Autodesk Inventor part; units mm, degrees
ref_plane "YZ Plane" through (0, 0, 0) normal (1, 0, 0) x (0, 1, 0)
ref_plane "XZ Plane" through (0, 0, 0) normal (0, 1, 0) x (-1, 0, 0)
ref_plane "XY Plane" through (0, 0, 0) normal (0, 0, 1) x (1, 0, 0)
sketch "Sketch1" plane through (0, 0, 0) normal (1, 0, 0) x (0, 1, 0)
  line L0 (0, 0) -> (6.52, 0)
  line L1 (6.52, 0) -> (6.52, -3)
  line L2 (6.52, -3) -> (0.86, -3)
  line L3 (0.86, -3) -> (0.86, -2.41)
  line L4 (0.86, -2.41) -> (0, -2.41)
  line L5 (0, -2.41) -> (0, 0)
  line L6 (0, -6.589) -> (-0.9134, -6.589)
  line L7 (0, 0) -> (-3.48, 0)
  line L8 (-3.48, 0) -> (-3.48, -3)
  line L9 (-3.48, -3) -> (0, -3)
  line L10 (0, -3) -> (0, 0)
  point P0 (-0.9134, 0)
  dimension "d1" = 3
  dimension "d2" = 5.66
  dimension "d6" = 0.86
  dimension "d8" = 10
  dimension "d9" = 2.41
revolve "Revolution1" add sketch "Sketch1" angle 360 about axis through (0, 0, 0) along (0, 1, 0)
sketch "Sketch2" plane through (0, -3.48, 0) normal (0, -1, 0) x (1, 0, 0)
  circle A0 centre (0, 0) radius 3
  line L0 (2.673, -0.4849) -> (-2.673, -0.4849)
  line L1 (-2.673, -0.4849) -> (-2.673, 0.4849)
  line L2 (-2.673, 0.4849) -> (2.673, 0.4849)
  line L3 (2.673, 0.4849) -> (2.673, -0.4849)
  line L4 (2.673, -0.4849) -> (-2.673, 0.4849) construction
  line L5 (-2.673, -0.4849) -> (2.673, 0.4849) construction
extrude "Extrusion1" add sketch "Sketch2" along normal blind 3 contours L0 L1 L2 L3
properties part number "00_IR_Laserdiode"
Check sheet for the modelled part. Datum: model origin and axes. Units: mm. A direction names the side the tool comes from. Round coordinates to 2 decimals unless told otherwise and drop trailing zeros. Loops run counter-clockwise (first coordinate to the right, second up) from the corner with the lowest first, then second, coordinate; pieces in that order, holes last.
1. Sectioned sample at A-A on x = 0. Record the boundary of the cut face in (y, z).
2. Sectioned sample at C-C on y = 3.5. Record the boundary of the cut face in (x, z), and give its area (3 significant figures).
3. Sectioned sample at D-D on z = -2. Record the boundary of the cut face in (x, y), and give its area (3 significant figures).
4. Scan lines: probe 1 along Y at (x, z) = (1.7, 2.3); probe 2 along Y at (x, z) = (0.8, 0.9); probe 3 along Z at (x, y) = (-2, -5.25). Record each from-to range of solid material in increasing order.
5. Sectioned sample at B-B on z = 0. Record the boundary of the cut face in (x, y).
6. Mould release check, pull along Y, two halves, no side actions. Record for faces 1 (the flat face through (0, -5, 0.485)), 2 (the flat face through (0, 6.52, 0)), 3 (the cylindrical face through (-2.353, 0.424, 0.522)): released by +Y, released by -Y, zero draft, split by the parting line, or undercut.
7. Gauge pin test, flat ends, axial feed: pin 1 Ø1.1 at (y, z) = (-5, 0) entering from +X; pin 2 Ø0.9 at (x, y) = (0.5, -5) entering from +Z; pin 3 Ø2.5 at (x, y) = (-1, -4.5) entering from -Z. Record the tip position at first contact, or that the pin passes through.
8. Set-up check for faces 4 (the cylindrical face through (0, 4, 3)), 5 (the flat face through (0, -6.48, 0)), 6 (the flat face through (2.673, -5, 0)), 7 (the flat face through (-2.673, -5, 0)), 8 (the flat face through (0, -5, -0.485)): record each of +Z, -Z, +X, -X, +Y, -Y from which the full face is reachable in a straight line by a thin tool's end or side.
Recorded:
1. outline: (-6.48, -0.48) - (-3.48, -0.48) - (-3.48, -3) - (0, -3) - (0, -2.41) - (0.86, -2.41) - (0.86, -3) - (6.52, -3) - (6.52, 3) - (0.86, 3) - (0.86, 2.41) - (0, 2.41) - (0, 3) - (-3.48, 3) - (-3.48, 0.48) - (-6.48, 0.48) - close
2. outline: circle Ø6 at (0, 0)
2. area: 28.3 mm2
3. outline: (-2.24, -3.48) - (2.24, -3.48) - (2.24, 0) - (1.34, 0) - (1.34, 0.86) - (2.24, 0.86) - (2.24, 6.52) - (-2.24, 6.52) - (-2.24, 0.86) - (-1.34, 0.86) - (-1.34, 0) - (-2.24, 0) - close
3. area: 43.2 mm2
4. probe 1: y = -3.48 to 0, 0.86 to 6.52
4. probe 2: y = -3.48 to 6.52
4. probe 3: z = -0.48 to 0.48
5. outline: (-3, -3.48) - (-2.67, -3.48) - (-2.67, -6.48) - (2.67, -6.48) - (2.67, -3.48) - (3, -3.48) - (3, 0) - (2.41, 0) - (2.41, 0.86) - (3, 0.86) - (3, 6.52) - (-3, 6.52) - (-3, 0.86) - (-2.41, 0.86) - (-2.41, 0) - (-3, 0) - close
6. face 1: zero draft
6. face 2: released by +Y
6. face 3: undercut
7. pin 1: stops at x = 2.67
7. pin 2: stops at z = 0.48
7. pin 3: stops at z = -2.99
8. face 4: +Y, -Y
8. face 5: +Z, -Z, +X, -X, -Y
8. face 6: +Z, -Z, +X, -Y
8. face 7: +Z, -Z, -X, -Y
8. face 8: -Z, +X, -X, -Y
